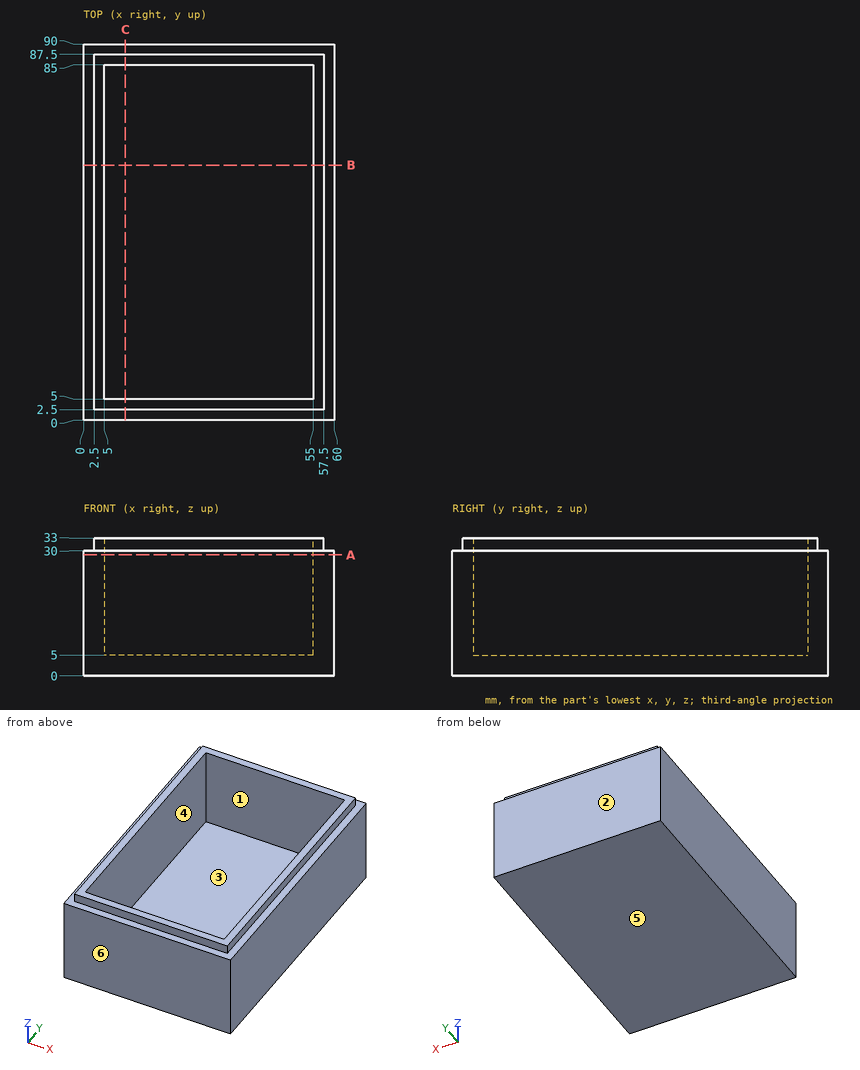
Input: dimensioned drawing with shaded views. Units: mm. Origin: part minimum x, y, z. A direction names the side the tool comes from. Round coordinates to 2 decimals unless told otherwise and drop trailing zeros. Loops run counter-clockwise (first coordinate to the right, second up) from the corner with the lowest first, then second, coordinate; pieces in that order, holes last. Notation, with made-up numbers: (74, 4) -> (113, 4) arc R19 ccw to (113, 28) -> close; hole circle Ø4 at (-40, 7). An arc over 180 degrees is marked (long way). Use one line per item in the form item = value. Start each with the question number.
1) Draft query along Y for the marked faces 3, 4, 5 and 6. Return one class per face: released by +Y, released by -Y, zero draft, split by the parting line, or undercut.
2) First-contact query: P1, Ø2.5, axis at x = 37.5, z = 32, coming from the -Y side; P2, Ø1, axis at x = 28.5, y = 77, coming from the +Z side; P3, Ø1.5, axis at x = 23, z = 31, coming from the +Y side. Flat tips, straight axial feed; report the tip coordinate or a pass-through.
3) Line query: L1, parallel to X at y = 57.5, z = 21; L2, parallel to X at y = 52, z = 31.5; L3, parallel to Y at x = 40, z = 17. Output: solid intervals per line, ascending.
4) Access query for the marked faces 1 and 2. Directions: +Z, -Z, +X, -X, +Y, -Y. A direction counts if a zero-diameter tool reaches every point of the face in a straight line with its end or side. Return the directions, or none.
5) Section A-A on z = 29. Output: boundary loops of the cut face in (x, y).
6) Section C-C on x = 10. Output: boundary loops of the cut face in (y, z).
7) Section B-B on y = 61. Output: boundary loops of the cut face in (x, z), then the cut area to 3 significant figures.
Response:
q1.face_3 = undercut
q1.face_4 = undercut
q1.face_5 = zero draft
q1.face_6 = released by -Y
q2.P1 = 2.5
q2.P2 = 5
q2.P3 = 87.5
q3.L1 = 0 to 5, 55 to 60
q3.L2 = 2.5 to 5, 55 to 57.5
q3.L3 = 0 to 5, 85 to 90
q4.face_1 = +Z
q4.face_2 = +Z, -Z, +X, -X, +Y
q5.outline = (0, 0) -> (60, 0) -> (60, 90) -> (0, 90) -> close; hole (5, 5) -> (55, 5) -> (55, 85) -> (5, 85) -> close
q6.outline = (0, 0) -> (90, 0) -> (90, 30) -> (87.5, 30) -> (87.5, 33) -> (85, 33) -> (85, 5) -> (5, 5) -> (5, 33) -> (2.5, 33) -> (2.5, 30) -> (0, 30) -> close
q7.outline = (0, 0) -> (60, 0) -> (60, 30) -> (57.5, 30) -> (57.5, 33) -> (55, 33) -> (55, 5) -> (5, 5) -> (5, 33) -> (2.5, 33) -> (2.5, 30) -> (0, 30) -> close
q7.area = 565 mm^2
